```python
from build123d import *

# Parameters (mm, degrees)
F0_R     = 1.5
F1_DEPTH = 3


with BuildPart() as f1:
    # F0 (on Top) → F1 (new body)
    with BuildSketch(Plane.XY):
        with BuildLine():
            ThreePointArc((0, 3), (0.87868, 0.87868), (3, 0))
            Line((3, 0), (95, 0))
            ThreePointArc((95, 0), (97.12132, 0.87868), (98, 3))
            Line((98, 3), (98, 8))
            ThreePointArc((98, 8), (97.707107, 8.707107), (97, 9))
            Line((97, 9), (77.5, 9))
            ThreePointArc((77.5, 9), (76.792893, 9.292893), (76.5, 10))
            Line((76.5, 10), (76.5, 24.5))
            ThreePointArc((76.5, 24.5), (76.792893, 25.207107), (77.5, 25.5))
            Line((77.5, 25.5), (97, 25.5))
            ThreePointArc((97, 25.5), (97.707107, 25.792893), (98, 26.5))
            Line((98, 26.5), (98, 28))
            ThreePointArc((98, 28), (97.707107, 28.707107), (97, 29))
            Line((97, 29), (82, 29))
            ThreePointArc((82, 29), (81.292893, 29.292893), (81, 30))
            Line((81, 30), (81, 42))
            ThreePointArc((81, 42), (81.292893, 42.707107), (82, 43))
            Line((82, 43), (97, 43))
            ThreePointArc((97, 43), (97.707107, 43.292893), (98, 44))
            Line((98, 44), (98, 46))
            ThreePointArc((98, 46), (97.707107, 46.707107), (97, 47))
            Line((97, 47), (82, 47))
            ThreePointArc((82, 47), (81.292893, 47.292893), (81, 48))
            Line((81, 48), (81, 60))
            ThreePointArc((81, 60), (81.292893, 60.707107), (82, 61))
            Line((82, 61), (97, 61))
            ThreePointArc((97, 61), (97.707107, 61.292893), (98, 62))
            Line((98, 62), (98, 67))
            ThreePointArc((98, 67), (97.12132, 69.12132), (95, 70))
            Line((95, 70), (73.5, 70))
            ThreePointArc((73.5, 70), (72.085786, 69.414214), (71.5, 68))
            Line((71.5, 68), (71.5, 57))
            ThreePointArc((71.5, 57), (70.914214, 55.585786), (69.5, 55))
            Line((69.5, 55), (18.5, 55))
            ThreePointArc((18.5, 55), (17.085786, 55.585786), (16.5, 57))
            Line((16.5, 57), (16.5, 68))
            ThreePointArc((16.5, 68), (15.914214, 69.414214), (14.5, 70))
            Line((14.5, 70), (3, 70))
            ThreePointArc((3, 70), (0.87868, 69.12132), (0, 67))
            Line((0, 67), (0, 3))
        make_face()
        with Locations((3, 3)):
            Circle(F0_R, mode=Mode.SUBTRACT)
        with Locations((73, 3)):
            Circle(F0_R, mode=Mode.SUBTRACT)
        with Locations((95, 3)):
            Circle(F0_R, mode=Mode.SUBTRACT)
        with Locations((3, 67)):
            Circle(F0_R, mode=Mode.SUBTRACT)
        with Locations((95, 67)):
            Circle(F0_R, mode=Mode.SUBTRACT)
    extrude(amount=F1_DEPTH)


solid = f1.part
```
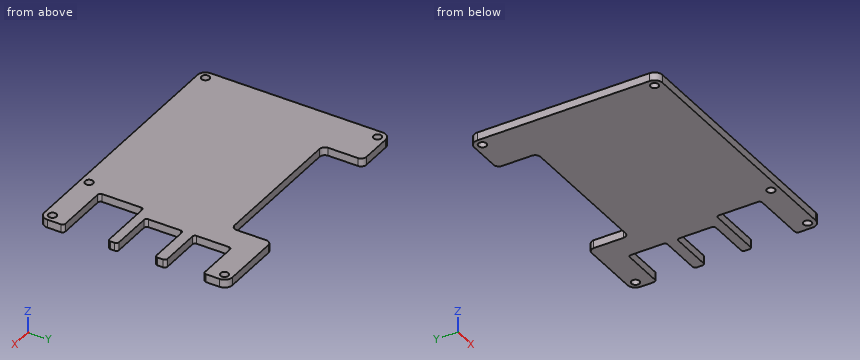
For this review, take the finished solid that the model builds, in its own axes (mm). Round coordinates to 2 decimals unless told otherwise and drop trailing zeros. Write each loop counter-clockwise with the first axis right and the second up, starting at its lowest first coordinate (ties: lowest second). Pieces come first, ordered by that corner, then holes. Notation, with made-up numbers: M -15.5,-0.5 L 21.5,-0.5 A18 ccw 21.5,23.5 Z; hole C 76,-26 d11. An arc over 180 degrees is marked long. One line per item, written item: value. Start each with the question number.
(1) Insertion check: pin 1 (0.9 mm diameter, centred on y = 56.5, z = 1.5, fed in from +X); pin 2 (5 mm diameter, centred on x = 95, y = 3, fed in from +Z); pin 3 (1.5 mm diameter, centred on y = 20.5, z = 1, fed in from +X). Each pin has a flat end and moves straight along its axis. Give the tip position at first contact, or say it passes through.
(2) We need section D-D (x = 28). Give the boundary of the cut face in (y, z).
(3) We need section A-A (x = 84.5). Give the boundary of the cut face in (y, z), and give its area (3 significant figures).
(4) We need section C-C (y = 38). Give the boundary of the cut face in (x, z).
(5) Wall thickness on line 1 (Y direction, x = 95, z = 1.5); line 2 (Y direction, x = 3, z = 1.55); line 3 (Y direction, x = 87.5, z = 0.9): over which ranges is each line inside the solid? List them lowest first.
(6) We need section B-B (z = 1.85). Count the separate pieces of the cut face and the enclosed holes in it, and give its area (3 significant figures).
Result:
1. pin 1: x = 81
1. pin 2: z = 3
1. pin 3: x = 76.5
2. outline: M 0,0 L 55,0 L 55,3 L 0,3 Z
3. outline: M 0,0 L 9,0 L 9,3 L 0,3 Z; M 25.5,0 L 29,0 L 29,3 L 25.5,3 Z; M 43,0 L 47,0 L 47,3 L 43,3 Z; M 61,0 L 70,0 L 70,3 L 61,3 Z
3. area: 76.5 mm²
4. outline: M 0,0 L 81,0 L 81,3 L 0,3 Z
5. line 1: 0 to 1.5, 4.5 to 9, 25.5 to 29, 43 to 47, 61 to 65.5, 68.5 to 70
5. line 2: 0 to 1.5, 4.5 to 65.5, 68.5 to 70
5. line 3: 0 to 9, 25.5 to 29, 43 to 47, 61 to 70
6. separate pieces: 1
6. enclosed holes: 5
6. area: 5,160 mm²
